Design review of the part built by this model. Coordinates are the model's own, in mm. Face numbers are marked on the shaded views. A direction names the side the tool comes from. Coordinates: 2 decimals unless noted, no trailing zeros. Write each loop counter-clockwise with the first axis right and the second up, starting at its lowest first coordinate (ties: lowest second). Pieces come first, ordered by that corner, then holes. Notation, with made-up numbers: (-7, 71) -> (23, 71) arc R28 cw to (23, 107) -> close; hole circle Ø5 at (43, 28). An arc over 180 degrees is marked (long way). Return JSON: item names as keys, results as strings. Group by question number.
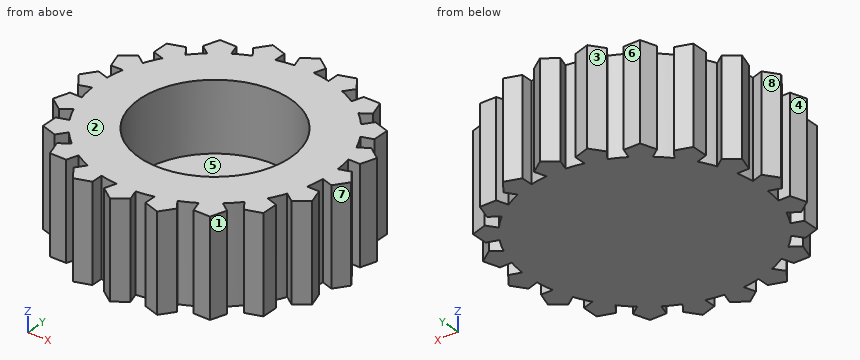
from build123d import *

# Parameters (mm, degrees)
BOSS_EXTRUDE1_OUTLINE_R = 5.5
BOSS_EXTRUDE1_DEPTH     = 7
SKETCH1_3_R             = 5.5
BOSS_EXTRUDE2_DEPTH     = 2


# Read off the part's stored shape, not the designer's step: Boss-Extrude1
with BuildPart() as part:
    # Boss-Extrude1 outline → Boss-Extrude1 (new body)
    with BuildSketch(Plane.XY):
        with BuildLine():
            Line((-0.970820393, 9.294657697), (-0.703154307, 8.470866191))
            ThreePointArc((-0.703154307, 8.470866191), (-1.329692953, 8.395350895), (-1.948902124, 8.27355912))
            Line((-1.948902124, 8.27355912), (-1.948902124, 9.13974477))
            Line((-1.948902124, 9.13974477), (-3.090169944, 9.510565163))
            Line((-3.090169944, 9.510565163), (-3.795512247, 8.53974477))
            Line((-3.795512247, 8.53974477), (-3.286381096, 7.838985859))
            ThreePointArc((-3.286381096, 7.838985859), (-3.858919248, 7.573555456), (-4.410186437, 7.266378437))
            Line((-4.410186437, 7.266378437), (-4.677852523, 8.090169944))
            Line((-4.677852523, 8.090169944), (-5.877852523, 8.090169944))
            Line((-5.877852523, 8.090169944), (-6.248672916, 6.948902124))
            Line((-6.248672916, 6.948902124), (-5.547914005, 6.439770973))
            ThreePointArc((-5.547914005, 6.439770973), (-6.01040764, 6.01040764), (-6.439770973, 5.547914005))
            Line((-6.439770973, 5.547914005), (-6.948902124, 6.248672916))
            Line((-6.948902124, 6.248672916), (-8.090169944, 5.877852523))
            Line((-8.090169944, 5.877852523), (-8.090169944, 4.677852523))
            Line((-8.090169944, 4.677852523), (-7.266378437, 4.410186437))
            ThreePointArc((-7.266378437, 4.410186437), (-7.573555456, 3.858919248), (-7.838985859, 3.286381096))
            Line((-7.838985859, 3.286381096), (-8.53974477, 3.795512246))
            Line((-8.53974477, 3.795512246), (-9.510565163, 3.090169944))
            Line((-9.510565163, 3.090169944), (-9.13974477, 1.948902124))
            Line((-9.13974477, 1.948902124), (-8.27355912, 1.948902124))
            ThreePointArc((-8.27355912, 1.948902124), (-8.395350895, 1.329692953), (-8.470866191, 0.703154307))
            Line((-8.470866191, 0.703154307), (-9.294657697, 0.970820393))
            Line((-9.294657697, 0.970820393), (-10, 0))
            Line((-10, 0), (-9.294657697, -0.970820393))
            Line((-9.294657697, -0.970820393), (-8.470866191, -0.703154307))
            ThreePointArc((-8.470866191, -0.703154307), (-8.395350895, -1.329692953), (-8.27355912, -1.948902124))
            Line((-8.27355912, -1.948902124), (-9.13974477, -1.948902124))
            Line((-9.13974477, -1.948902124), (-9.510565163, -3.090169944))
            Line((-9.510565163, -3.090169944), (-8.53974477, -3.795512247))
            Line((-8.53974477, -3.795512247), (-7.838985859, -3.286381096))
            ThreePointArc((-7.838985859, -3.286381096), (-7.573555456, -3.858919248), (-7.266378437, -4.410186437))
            Line((-7.266378437, -4.410186437), (-8.090169944, -4.677852523))
            Line((-8.090169944, -4.677852523), (-8.090169944, -5.877852523))
            Line((-8.090169944, -5.877852523), (-6.948902124, -6.248672916))
            Line((-6.948902124, -6.248672916), (-6.439770973, -5.547914005))
            ThreePointArc((-6.439770973, -5.547914005), (-6.01040764, -6.01040764), (-5.547914005, -6.439770973))
            Line((-5.547914005, -6.439770973), (-6.248672916, -6.948902124))
            Line((-6.248672916, -6.948902124), (-5.877852523, -8.090169944))
            Line((-5.877852523, -8.090169944), (-4.677852523, -8.090169944))
            Line((-4.677852523, -8.090169944), (-4.410186437, -7.266378437))
            ThreePointArc((-4.410186437, -7.266378437), (-3.858919248, -7.573555456), (-3.286381096, -7.838985859))
            Line((-3.286381096, -7.838985859), (-3.795512246, -8.53974477))
            Line((-3.795512246, -8.53974477), (-3.090169944, -9.510565163))
            Line((-3.090169944, -9.510565163), (-1.948902124, -9.13974477))
            Line((-1.948902124, -9.13974477), (-1.948902124, -8.27355912))
            ThreePointArc((-1.948902124, -8.27355912), (-1.329692953, -8.395350895), (-0.703154307, -8.470866191))
            Line((-0.703154307, -8.470866191), (-0.970820393, -9.294657697))
            Line((-0.970820393, -9.294657697), (0, -10))
            Line((0, -10), (0.970820393, -9.294657697))
            Line((0.970820393, -9.294657697), (0.703154307, -8.470866191))
            ThreePointArc((0.703154307, -8.470866191), (1.329692953, -8.395350895), (1.948902124, -8.27355912))
            Line((1.948902124, -8.27355912), (1.948902124, -9.13974477))
            Line((1.948902124, -9.13974477), (3.090169944, -9.510565163))
            Line((3.090169944, -9.510565163), (3.795512247, -8.53974477))
            Line((3.795512247, -8.53974477), (3.286381096, -7.838985859))
            ThreePointArc((3.286381096, -7.838985859), (3.858919248, -7.573555456), (4.410186437, -7.266378437))
            Line((4.410186437, -7.266378437), (4.677852523, -8.090169944))
            Line((4.677852523, -8.090169944), (5.877852523, -8.090169944))
            Line((5.877852523, -8.090169944), (6.248672916, -6.948902124))
            Line((6.248672916, -6.948902124), (5.547914005, -6.439770973))
            ThreePointArc((5.547914005, -6.439770973), (6.01040764, -6.01040764), (6.439770973, -5.547914005))
            Line((6.439770973, -5.547914005), (6.948902124, -6.248672916))
            Line((6.948902124, -6.248672916), (8.090169944, -5.877852523))
            Line((8.090169944, -5.877852523), (8.090169944, -4.677852523))
            Line((8.090169944, -4.677852523), (7.266378437, -4.410186437))
            ThreePointArc((7.266378437, -4.410186437), (7.573555456, -3.858919248), (7.838985859, -3.286381096))
            Line((7.838985859, -3.286381096), (8.53974477, -3.795512246))
            Line((8.53974477, -3.795512246), (9.510565163, -3.090169944))
            Line((9.510565163, -3.090169944), (9.13974477, -1.948902124))
            Line((9.13974477, -1.948902124), (8.27355912, -1.948902124))
            ThreePointArc((8.27355912, -1.948902124), (8.395350895, -1.329692953), (8.470866191, -0.703154307))
            Line((8.470866191, -0.703154307), (9.294657697, -0.970820393))
            Line((9.294657697, -0.970820393), (10, 0))
            Line((10, 0), (9.294657697, 0.970820393))
            Line((9.294657697, 0.970820393), (8.470866191, 0.703154307))
            ThreePointArc((8.470866191, 0.703154307), (8.395350895, 1.329692953), (8.27355912, 1.948902124))
            Line((8.27355912, 1.948902124), (9.13974477, 1.948902124))
            Line((9.13974477, 1.948902124), (9.510565163, 3.090169944))
            Line((9.510565163, 3.090169944), (8.53974477, 3.795512247))
            Line((8.53974477, 3.795512247), (7.838985859, 3.286381096))
            ThreePointArc((7.838985859, 3.286381096), (7.573555456, 3.858919248), (7.266378437, 4.410186437))
            Line((7.266378437, 4.410186437), (8.090169944, 4.677852523))
            Line((8.090169944, 4.677852523), (8.090169944, 5.877852523))
            Line((8.090169944, 5.877852523), (6.948902124, 6.248672916))
            Line((6.948902124, 6.248672916), (6.439770973, 5.547914005))
            ThreePointArc((6.439770973, 5.547914005), (6.01040764, 6.01040764), (5.547914005, 6.439770973))
            Line((5.547914005, 6.439770973), (6.248672916, 6.948902124))
            Line((6.248672916, 6.948902124), (5.877852523, 8.090169944))
            Line((5.877852523, 8.090169944), (4.677852523, 8.090169944))
            Line((4.677852523, 8.090169944), (4.410186437, 7.266378437))
            ThreePointArc((4.410186437, 7.266378437), (3.858919248, 7.573555456), (3.286381096, 7.838985859))
            Line((3.286381096, 7.838985859), (3.795512247, 8.53974477))
            Line((3.795512247, 8.53974477), (3.090169944, 9.510565163))
            Line((3.090169944, 9.510565163), (1.948902124, 9.13974477))
            Line((1.948902124, 9.13974477), (1.948902124, 8.27355912))
            ThreePointArc((1.948902124, 8.27355912), (1.329692953, 8.395350895), (0.703154307, 8.470866191))
            Line((0.703154307, 8.470866191), (0.970820393, 9.294657697))
            Line((0.970820393, 9.294657697), (0, 10))
            Line((0, 10), (-0.970820393, 9.294657697))
        make_face()
        Circle(BOSS_EXTRUDE1_OUTLINE_R, mode=Mode.SUBTRACT)
    extrude(amount=BOSS_EXTRUDE1_DEPTH)

    # Sketch1<3> → Boss-Extrude2 (add)
    with BuildSketch(Plane.XY):
        Circle(SKETCH1_3_R)
    extrude(amount=BOSS_EXTRUDE2_DEPTH)


solid = part.part
Q1. Wall thickness on L1, parallel to Y at x = 9, z = 1.75; L2, parallel to Y at x = -7.5, z = 6.5; L3, parallel to X at y = 1.75, z = 3.5: over which ranges is each line inside the solid? List them lowest first.
Q2. For the marked faces 5, 6, 7 and 8, list the 3-axis set-ups (+Z, -Z, +X, -X, +Y, -Y) from which the entire face can be reached by the end or side of a thin tool; tool diameter is ignored.
Q3. We need section A-A on x = 1.25. Write out the cut boundary in (y, z), plus the area to 3 significant figures.
Q4. We need section B-B on y = -5. Write out the cut boundary in (x, z).
Q5. The part is to be moulded in two halves that separate along Y. For the marked faces 1, 2, 3 and 4, say which applies: +Y half, -Y half, draft (parallel to the pull), parting line (faces both ways), or undercut.
Q6. For P1, Ø1.3, axis at x = -5.5, z = 5, coming from the +Y side; P2, Ø0.7, axis at y = -8.5, z = 5, coming from the -X side; P3, Ø5.5, axis at x = -1, y = -2, coming from the +Z side, all flat-tipped, find the tip position at first contact; note any pin that passes through.
Findings below:
{
 "1": {"L1": "y = -3.46 to -1.95, -0.88 to 0.88, 1.95 to 3.46", "L2": "y = -6.07 to -4.49, -4 to 4, 4.49 to 6.07", "L3": "x = -8.32 to -5.21, 5.21 to 8.32"},
 "2": {"face 5": "+Z", "face 6": "+Z, -Z, -X, +Y", "face 7": "+Z, -Z, +X", "face 8": "+Z, -Z, -X"},
 "3": {"outline": "(-8.41, 0) -> (8.41, 0) -> (8.41, 7) -> (5.36, 7) -> (5.36, 2) -> (-5.36, 2) -> (-5.36, 7) -> (-8.41, 7) -> close", "area": "64.1 mm^2"},
 "4": {"outline": "(-8.09, 0) -> (8.09, 0) -> (8.09, 7) -> (2.29, 7) -> (2.29, 2) -> (-2.29, 2) -> (-2.29, 7) -> (-8.09, 7) -> close"},
 "5": {"face 1": "-Y half", "face 2": "draft", "face 3": "+Y half", "face 4": "undercut"},
 "6": {"P1": "stops at y = 8.09", "P2": "stops at x = -3.8", "P3": "stops at z = 2"}
}
